Source: CAD feature listing. Evaluate the final solid. Frame: model axes, mm. A direction names the side the tool comes from. Give positions to 0.01 mm unless a question says otherwise; leave off trailing zeros. Order: outer loops, then holes, each group sorted by start corner. A loop starts at its lowest first (then second) coordinate and runs counter-clockwise, first axis right, second up. Notation, with made-up numbers: M 12.25,-35 L 19.25,-35 A9 ccw 19.25,-20 Z; hole C 64.5,83 d6. An arc over 180 degrees is marked long. Return JSON: item names as keys, results as strings.
from build123d import *

# Parameters (mm, degrees)
SKETCH_1_W          = 20
SKETCH_1_H          = 10
SKETCH_1_W_2        = 16
SKETCH_1_H_2        = 6
EXTRUDE_1_DEPTH     = 140
SKETCH_3_R          = 1.5
CUT_EXTRUDE_1_DEPTH = 142.509716981


with BuildPart() as part:
    # 草图1 → 凸台-拉伸1 (new, symmetric)
    with BuildSketch(Plane(origin=(0, 0, 0), x_dir=(1, 0, 0), z_dir=(0, 1, 0))):
        Rectangle(SKETCH_1_W, SKETCH_1_H)
        Rectangle(SKETCH_1_W_2, SKETCH_1_H_2, mode=Mode.SUBTRACT)
    extrude(amount=EXTRUDE_1_DEPTH, both=True)

    # 草图3 → 切除-拉伸1 (cut, through all)
    with BuildSketch(Plane(origin=(10, 0, 0), x_dir=(0, 0, -1), z_dir=(1, 0, 0))):
        with Locations((0, 130)):
            Circle(SKETCH_3_R)
        with Locations((0, 120)):
            Circle(SKETCH_3_R)
        with Locations((0, 110)):
            Circle(SKETCH_3_R)
        with Locations((0, -110)):
            Circle(SKETCH_3_R)
        with Locations((0, -120)):
            Circle(SKETCH_3_R)
        with Locations((0, -130)):
            Circle(SKETCH_3_R)
    extrude(amount=-CUT_EXTRUDE_1_DEPTH, mode=Mode.SUBTRACT)


solid = part.part
1. Draft query along Z for faces 1 (the face through (10, 2, 0)), 2 (the face through (0, 2, -3)), 3 (the face through (0, 2, -5)). Return one class per face: pulls with the +Z half, pulls with the -Z half, needs draft (parallel to the pull), parting line crosses it, or undercut.
Evaluation:
{"face 1": "needs draft", "face 2": "undercut", "face 3": "pulls with the -Z half"}
2. Section query C-C (z = 0). State how many separate pieces and enclosed holes the cut face has, then the cut area to 3 significant figures.
Evaluation:
{"separate pieces": "14", "enclosed holes": "0", "area": "1,050 mm^2"}
3. Section query B-B (y = -105.5). Return loops of the section in (x, z).
Evaluation:
{"outline": "M -10,-5 L 10,-5 L 10,5 L -10,5 Z; hole M -8,-3 L 8,-3 L 8,3 L -8,3 Z"}
4. Section query A-A (x = 0). Return loops of the section in (y, z).
Evaluation:
{"outline": "M -140,-5 L 140,-5 L 140,-3 L -140,-3 Z; M -140,3 L 140,3 L 140,5 L -140,5 Z"}
5. Set-up query: faces 4 (the face through (0, 2, 3)), 5 (the face through (-0.1, -140, -3.4)). Return all of +Z, -Z, +X, -X, +Y, -Y with unobstructed straight access to the full face (end or side cutting, diameter ignored); none if empty.
Evaluation:
{"face 4": "+Y, -Y", "face 5": "+Z, -Z, +X, -X, -Y"}
6. Ray query, probe 1 along X at (y, z) = (21.5, 0.25); probe 2 along Z at (x, y) = (4.25, -12.5); probe 3 along Z at (x, y) = (9.4, -130). Return the intervals inside material, ascending.
Evaluation:
{"probe 1": "x = -10 to -8, 8 to 10", "probe 2": "z = -5 to -3, 3 to 5", "probe 3": "z = -5 to -1.5, 1.5 to 5"}
